from build123d import *

# Parameters (mm, degrees)
BOSS_EXTRUDE1_DEPTH                   = 17.5
CUT_EXTRUDE1_DEPTH                    = 32
CUT_EXTRUDE2_DEPTH                    = 2
BOSS_EXTRUDE2_DEPTH                   = 2
CUT_EXTRUDE3_DEPTH                    = 11
CIRPATTERN1_COUNT                     = 4
SKETCH6_R                             = 2
CUT_EXTRUDE4_DEPTH                    = 174.692256592
CIRPATTERN2_COUNT                     = 4
TAP_DRILL_FOR_M3_TAP1_D               = 2.5
TAP_DRILL_FOR_M3_TAP1_DEPTH           = 20
TAP_DRILL_FOR_M3_TAP1_ON_FACE_2_D     = 2.5
TAP_DRILL_FOR_M3_TAP1_ON_FACE_2_DEPTH = 20
TAP_DRILL_FOR_M3_TAP1_ON_FACE_3_D     = 2.5
TAP_DRILL_FOR_M3_TAP1_ON_FACE_3_DEPTH = 20
TAP_DRILL_FOR_M3_TAP1_ON_FACE_4_D     = 2.5
TAP_DRILL_FOR_M3_TAP1_ON_FACE_4_DEPTH = 20
F_3_0_3_DIAMETER_HOLE1_D              = 3
F_3_0_3_DIAMETER_HOLE1_DEPTH          = 20
F_3_0_3_DIAMETER_HOLE1_TIP            = 0.901290929
CUT_EXTRUDE5_REACH                    = 253.357
SKETCH16_R                            = 3.5
CUT_EXTRUDE6_DEPTH                    = 10
M3X0_5_TAPPED_HOLE1_D                 = 2.5
M3X0_5_TAPPED_HOLE1_DEPTH             = 5
M3X0_5_TAPPED_HOLE1_TIP               = 0.751075774


with BuildPart() as part:
    # Sketch1 → Boss-Extrude1 (new, symmetric)
    with BuildSketch(Plane(origin=(0, 0, 0), x_dir=(1, 0, 0), z_dir=(0, 1, 0))):
        with BuildLine():
            ThreePointArc((-110, 100), (-102.928932188, 97.071067812), (-100, 90))
            Line((-100, 90), (-100, -90))
            ThreePointArc((-100, -90), (-102.928932188, -97.071067812), (-110, -100))
            Line((-110, -100), (-120, -100))
            Line((-120, -100), (-120, -120))
            Line((-120, -120), (-100, -120))
            Line((-100, -120), (-100, -110))
            ThreePointArc((-100, -110), (-97.071067812, -102.928932188), (-90, -100))
            Line((-90, -100), (90, -100))
            ThreePointArc((90, -100), (97.071067812, -102.928932188), (100, -110))
            Line((100, -110), (100, -120))
            Line((100, -120), (120, -120))
            Line((120, -120), (120, -100))
            Line((120, -100), (110, -100))
            ThreePointArc((110, -100), (102.928932188, -97.071067812), (100, -90))
            Line((100, -90), (100, 90))
            ThreePointArc((100, 90), (102.928932188, 97.071067812), (110, 100))
            Line((110, 100), (120, 100))
            Line((120, 100), (120, 120))
            Line((120, 120), (100, 120))
            Line((100, 120), (100, 110))
            ThreePointArc((100, 110), (97.071067812, 102.928932188), (90, 100))
            Line((90, 100), (-90, 100))
            ThreePointArc((-90, 100), (-97.071067812, 102.928932188), (-100, 110))
            Line((-100, 110), (-100, 120))
            Line((-100, 120), (-120, 120))
            Line((-120, 120), (-120, 100))
            Line((-120, 100), (-110, 100))
        make_face()
    extrude(amount=BOSS_EXTRUDE1_DEPTH, both=True)

    # Sketch2 → Cut-Extrude1 (cut)
    with BuildSketch(Plane(origin=(0, 17.5, 0), x_dir=(1, 0, 0), z_dir=(0, 1, 0))):
        with BuildLine():
            Line((-88, 98), (88, 98))
            ThreePointArc((88, 98), (95.071067812, 95.071067812), (98, 88))
            Line((98, 88), (98, -88))
            ThreePointArc((98, -88), (95.071067812, -95.071067812), (88, -98))
            Line((88, -98), (-88, -98))
            ThreePointArc((-88, -98), (-95.071067812, -95.071067812), (-98, -88))
            Line((-98, -88), (-98, 88))
            ThreePointArc((-98, 88), (-95.071067812, 95.071067812), (-88, 98))
        make_face()
    extrude(amount=-CUT_EXTRUDE1_DEPTH, mode=Mode.SUBTRACT)

    # Sketch3 → Cut-Extrude2 (cut)
    with BuildSketch(Plane(origin=(0, -14.5, 0), x_dir=(1, 0, 0), z_dir=(0, 1, 0))):
        with BuildLine():
            Line((-88, -96), (88, -96))
            ThreePointArc((88, -96), (93.656854249, -93.656854249), (96, -88))
            Line((96, -88), (96, 88))
            ThreePointArc((96, 88), (93.656854249, 93.656854249), (88, 96))
            Line((88, 96), (-88, 96))
            ThreePointArc((-88, 96), (-93.656854249, 93.656854249), (-96, 88))
            Line((-96, 88), (-96, -88))
            ThreePointArc((-96, -88), (-93.656854249, -93.656854249), (-88, -96))
        make_face()
    extrude(amount=-CUT_EXTRUDE2_DEPTH, mode=Mode.SUBTRACT)

    # Sketch4 → Boss-Extrude2 (add)
    with BuildSketch(Plane.XZ.offset(17.5)):
        with BuildLine():
            Line((-88, -98), (88, -98))
            ThreePointArc((88, -98), (95.071067812, -95.071067812), (98, -88))
            Line((98, -88), (98, 88))
            ThreePointArc((98, 88), (95.071067812, 95.071067812), (88, 98))
            Line((88, 98), (-88, 98))
            ThreePointArc((-88, 98), (-95.071067812, 95.071067812), (-98, 88))
            Line((-98, 88), (-98, -88))
            ThreePointArc((-98, -88), (-95.071067812, -95.071067812), (-88, -98))
        make_face()
    extrude(amount=BOSS_EXTRUDE2_DEPTH)

    # Sketch5 → Cut-Extrude3 (cut)
    with BuildSketch(Plane(origin=(0, -5.5, 0), x_dir=(1, 0, 0), z_dir=(0, 1, 0))):
        Polygon((-120, 100.61731573), (-100.61731573, 120), (-120, 120), align=None)
    cut_extrude3 = extrude(amount=CUT_EXTRUDE3_DEPTH, mode=Mode.SUBTRACT)

    # CirPattern1: Cut-Extrude3 ×4 about axis
    cirpattern1_axis = Axis((0, 0, 0), (0, 1, 0))
    for i in range(1, CIRPATTERN1_COUNT):
        add(cut_extrude3.rotate(cirpattern1_axis, i * 360 / CIRPATTERN1_COUNT), mode=Mode.SUBTRACT)

    # Sketch6 → Cut-Extrude4 (cut, through all)
    with BuildSketch(Plane(origin=(0, 17.5, 0), x_dir=(1, 0, 0), z_dir=(0, 1, 0))):
        with Locations(Location((-112.493820949, 112.493820949, 0), (0, 0, 270))):
            Circle(SKETCH6_R)
    cut_extrude4 = extrude(amount=-CUT_EXTRUDE4_DEPTH, mode=Mode.SUBTRACT)

    # CirPattern2: Cut-Extrude4 ×4 about axis
    cirpattern2_axis = Axis((0, 0, 0), (0, 1, 0))
    for i in range(1, CIRPATTERN2_COUNT):
        add(cut_extrude4.rotate(cirpattern2_axis, i * 360 / CIRPATTERN2_COUNT), mode=Mode.SUBTRACT)

    # Tap Drill for M3 Tap1
    with Locations(Plane(origin=(116, 11.5, -120), x_dir=(-1, 0, 0), z_dir=(0, 0, -1))):
        with Locations((0, 0), (232, -23)):
            Hole(TAP_DRILL_FOR_M3_TAP1_D / 2, depth=TAP_DRILL_FOR_M3_TAP1_DEPTH)

    # Tap Drill for M3 Tap1 on face 2
    with Locations(Plane(origin=(-120, 11.5, -116), x_dir=(0, 0, -1), z_dir=(-1, 0, 0))):
        with Locations((0, 0), (-232, 23)):
            Hole(TAP_DRILL_FOR_M3_TAP1_ON_FACE_2_D / 2, depth=TAP_DRILL_FOR_M3_TAP1_ON_FACE_2_DEPTH)

    # Tap Drill for M3 Tap1 on face 3
    with Locations(Plane(origin=(-116, 11.5, 120), x_dir=(1, 0, 0), z_dir=(0, 0, 1))):
        with Locations((0, 0), (232, -23)):
            Hole(TAP_DRILL_FOR_M3_TAP1_ON_FACE_3_D / 2, depth=TAP_DRILL_FOR_M3_TAP1_ON_FACE_3_DEPTH)

    # Tap Drill for M3 Tap1 on face 4
    with Locations(Plane(origin=(120, 11.5, 116), x_dir=(0, 0, 1), z_dir=(1, 0, 0))):
        with Locations((0, 0), (-232, 23)):
            Hole(TAP_DRILL_FOR_M3_TAP1_ON_FACE_4_D / 2, depth=TAP_DRILL_FOR_M3_TAP1_ON_FACE_4_DEPTH)

    # Ø3.0 (3) Diameter Hole1
    with Locations(Plane(origin=(0, 0, 0), x_dir=(1, 0, 0), z_dir=(0, 1, 0))):
        with Locations((-83, 89), (0, 89), (83, 89), (87, 1), (-87, 1), (-87, -87), (0, -87), (87, -87)):
            Hole(F_3_0_3_DIAMETER_HOLE1_D / 2, depth=F_3_0_3_DIAMETER_HOLE1_DEPTH)
            with Locations((0, 0, -(F_3_0_3_DIAMETER_HOLE1_DEPTH + F_3_0_3_DIAMETER_HOLE1_TIP / 2))):  # 118° drill point
                Cone(0, F_3_0_3_DIAMETER_HOLE1_D / 2, F_3_0_3_DIAMETER_HOLE1_TIP, mode=Mode.SUBTRACT)

    # Sketch16 → Cut-Extrude5 (cut, up to next)
    with BuildSketch(Plane(origin=(0, 0, -100), x_dir=(-1, 0, 0), z_dir=(0, 0, -1)), mode=Mode.PRIVATE) as cut_extrude5_sk1:
        with Locations((0, 8.1)):
            Circle(SKETCH16_R)
    cut_extrude5_tool1 = extrude(cut_extrude5_sk1.sketch, amount=-CUT_EXTRUDE5_REACH, mode=Mode.PRIVATE) & part.part
    # Sketch16 → Cut-Extrude5 (cut, up to next)
    with BuildSketch(Plane(origin=(0, 0, -100), x_dir=(-1, 0, 0), z_dir=(0, 0, -1)), mode=Mode.PRIVATE) as cut_extrude5_sk2:
        with Locations((32.67, 8.1)):
            Circle(SKETCH16_R)
    cut_extrude5_tool2 = extrude(cut_extrude5_sk2.sketch, amount=-CUT_EXTRUDE5_REACH, mode=Mode.PRIVATE) & part.part
    # Sketch16 → Cut-Extrude5 (cut, up to next)
    with BuildSketch(Plane(origin=(0, 0, -100), x_dir=(-1, 0, 0), z_dir=(0, 0, -1)), mode=Mode.PRIVATE) as cut_extrude5_sk3:
        with Locations((65.34, 8.1)):
            Circle(SKETCH16_R)
    cut_extrude5_tool3 = extrude(cut_extrude5_sk3.sketch, amount=-CUT_EXTRUDE5_REACH, mode=Mode.PRIVATE) & part.part
    # Sketch16 → Cut-Extrude5 (cut, up to next)
    with BuildSketch(Plane(origin=(0, 0, -100), x_dir=(-1, 0, 0), z_dir=(0, 0, -1)), mode=Mode.PRIVATE) as cut_extrude5_sk4:
        with Locations((-32.67, 8.1)):
            Circle(SKETCH16_R)
    cut_extrude5_tool4 = extrude(cut_extrude5_sk4.sketch, amount=-CUT_EXTRUDE5_REACH, mode=Mode.PRIVATE) & part.part
    # Sketch16 → Cut-Extrude5 (cut, up to next)
    with BuildSketch(Plane(origin=(0, 0, -100), x_dir=(-1, 0, 0), z_dir=(0, 0, -1)), mode=Mode.PRIVATE) as cut_extrude5_sk5:
        with Locations((-65.34, 8.1)):
            Circle(SKETCH16_R)
    cut_extrude5_tool5 = extrude(cut_extrude5_sk5.sketch, amount=-CUT_EXTRUDE5_REACH, mode=Mode.PRIVATE) & part.part
    add(cut_extrude5_tool1.solids().sort_by_distance((0, 8.1, -100))[0], mode=Mode.SUBTRACT)
    add(cut_extrude5_tool2.solids().sort_by_distance((-32.67, 8.1, -100))[0], mode=Mode.SUBTRACT)
    add(cut_extrude5_tool3.solids().sort_by_distance((-65.34, 8.1, -100))[0], mode=Mode.SUBTRACT)
    add(cut_extrude5_tool4.solids().sort_by_distance((32.67, 8.1, -100))[0], mode=Mode.SUBTRACT)
    add(cut_extrude5_tool5.solids().sort_by_distance((65.34, 8.1, -100))[0], mode=Mode.SUBTRACT)

    # Sketch17 → Cut-Extrude6 (cut)
    with BuildSketch(Plane.XY.offset(100)):
        with BuildLine():
            Line((-51.97665364, 4.23), (-38.20334636, 4.23))
            ThreePointArc((-38.20334636, 4.23), (-35.598795254, 3.015477873), (-34.855, 0.239596196))
            Line((-34.855, 0.239596196), (-35.666104111, -4.360403804))
            ThreePointArc((-35.666104111, -4.360403804), (-36.828972599, -6.374551107), (-39.014450472, -7.17))
            Line((-39.014450472, -7.17), (-51.165549528, -7.17))
            ThreePointArc((-51.165549528, -7.17), (-53.351027401, -6.374551107), (-54.513895889, -4.360403804))
            Line((-54.513895889, -4.360403804), (-55.325, 0.239596196))
            ThreePointArc((-55.325, 0.239596196), (-54.581204746, 3.015477873), (-51.97665364, 4.23))
        make_face()
        with BuildLine():
            Line((16.271104111, -4.360403804), (15.46, 0.239596196))
            ThreePointArc((15.46, 0.239596196), (16.203795254, 3.015477873), (18.80834636, 4.23))
            Line((18.80834636, 4.23), (71.19165364, 4.23))
            ThreePointArc((71.19165364, 4.23), (73.796204746, 3.015477873), (74.54, 0.239596196))
            Line((74.54, 0.239596196), (73.728895889, -4.360403804))
            ThreePointArc((73.728895889, -4.360403804), (72.566027401, -6.374551107), (70.380549528, -7.17))
            Line((70.380549528, -7.17), (19.619450472, -7.17))
            ThreePointArc((19.619450472, -7.17), (17.433972599, -6.374551107), (16.271104111, -4.360403804))
        make_face()
    extrude(amount=-CUT_EXTRUDE6_DEPTH, mode=Mode.SUBTRACT)

    # M3x0.5 Tapped Hole1
    with Locations(Plane.XY.offset(100)):
        with Locations((-57.585, -1.47), (-32.595, -1.47), (13.25, -1.47), (76.75, -1.47)):
            Hole(M3X0_5_TAPPED_HOLE1_D / 2, depth=M3X0_5_TAPPED_HOLE1_DEPTH)
            with Locations((0, 0, -(M3X0_5_TAPPED_HOLE1_DEPTH + M3X0_5_TAPPED_HOLE1_TIP / 2))):  # 118° drill point
                Cone(0, M3X0_5_TAPPED_HOLE1_D / 2, M3X0_5_TAPPED_HOLE1_TIP, mode=Mode.SUBTRACT)


solid = part.part
CAD build for the part. Positions are in the model's coordinates, mm. A direction names the side the tool comes from. Coordinates: 2 decimals unless noted, no trailing zeros. Loops run counter-clockwise (first coordinate to the right, second up) from the corner with the lowest first, then second, coordinate; pieces in that order, holes last. Notation, with made-up numbers: (17, 81.5) -> (49, 81.5) arc R8 cw to (49, 96.5) -> close; hole circle Ø3 at (-40, -6.5). An arc over 180 degrees is marked (long way). One line per item, written item: value.
1. Pull direction Z, two halves, no side cores. Call faces 4 (the face through (115, 0, -100)), 5 (the face through (1, 2, 98)), 6 (the face through (-94.99, -18.49, 95.15)), 7 (the face through (115, 5.5, -113)): pulls with the +Z half, pulls with the -Z half, needs draft (parallel to the pull), parting line crosses it, or undercut.
Answers:
face 4: undercut
face 5: undercut
face 6: pulls with the +Z half
face 7: needs draft
2. Slice it at C-C on z = 31. Write the cut outline in (x, y), and give its area (3 significant figures).
Answers:
outline: (-100, -17.5) -> (-98, -17.5) -> (-98, -19.5) -> (98, -19.5) -> (98, -17.5) -> (100, -17.5) -> (100, 17.5) -> (98, 17.5) -> (98, -14.5) -> (96, -14.5) -> (96, -16.5) -> (-96, -16.5) -> (-96, -14.5) -> (-98, -14.5) -> (-98, 17.5) -> (-100, 17.5) -> close
area: 736 mm^2
3. Slice it at B-B on x = -65.34. Write the cut outline in (y, z), and give its area (3 significant figures).
Answers:
outline: (-19.5, -98) -> (-17.5, -98) -> (-17.5, -100) -> (4.6, -100) -> (4.6, -98) -> (-14.5, -98) -> (-14.5, -96) -> (-16.5, -96) -> (-16.5, 96) -> (-14.5, 96) -> (-14.5, 98) -> (17.5, 98) -> (17.5, 100) -> (-17.5, 100) -> (-17.5, 98) -> (-19.5, 98) -> close; (11.6, -100) -> (17.5, -100) -> (17.5, -98) -> (11.6, -98) -> close
area: 722 mm^2
4. Drill centre lines: line 1 (Z direction, x = 0, y = -18.1); line 2 (X direction, y = -17, z = -89); line 3 (Z direction, x = -4, y = -12.5). Where is each one in solid material? Low to high. Write a range as [from, to].
Answers:
line 1: z = [-98, -90.5], [-87.5, 85.5], [88.5, 98]
line 2: x = [-100, -84.5], [-81.5, -1.5], [1.5, 81.5], [84.5, 100]
line 3: z = [-100, -98], [98, 100]
5. Slice it at A-A on x = 65.34. Write the cut outline in (y, z).
Answers:
outline: (-19.5, -98) -> (-17.5, -98) -> (-17.5, -100) -> (4.6, -100) -> (4.6, -98) -> (-14.5, -98) -> (-14.5, -96) -> (-16.5, -96) -> (-16.5, 96) -> (-14.5, 96) -> (-14.5, 98) -> (-7.17, 98) -> (-7.17, 100) -> (-17.5, 100) -> (-17.5, 98) -> (-19.5, 98) -> close; (4.23, 98) -> (17.5, 98) -> (17.5, 100) -> (4.23, 100) -> close; (11.6, -100) -> (17.5, -100) -> (17.5, -98) -> (11.6, -98) -> close
6. Flat gauge pins, fed straight in: P1, Ø1, axis at x = 57, z = -87, coming from the +Y side; P2, Ø10, axis at x = -11, y = 13.5, coming from the +Z side; P3, Ø1.5, axis at y = -5.5, z = 87, coming from the -X side; P4, Ø4.5, axis at x = -112.49, z = 112.49, coming from the +Y side. Where does each tip first touch, or does it go through?
Answers:
P1: stops at y = -16.5
P2: stops at z = 100
P3: stops at x = -100
P4: stops at y = 17.5
7. Which spindle directions (+Z, -Z, +X, -X, +Y, -Y) get a long thin tool onto all of the face, cutting with end or side? Do faces 1 (the face through (-94.99, 1.72, 95.15)), 2 (the face through (-115, 0, 100)), 3 (the face through (100, 0, 1)). Say none if no direction does.
Answers:
face 1: +Y
face 2: -X, +Y, -Y
face 3: +X, +Y, -Y
